Check sheet for the modelled part. Datum: model origin and axes. Units: mm. A direction names the side the tool comes from. Coordinates: 2 decimals unless noted, no trailing zeros. Loops run counter-clockwise (first coordinate to the right, second up) from the corner with the lowest first, then second, coordinate; pieces in that order, holes last.
from build123d import *

# Parameters (mm, degrees)
EXTRUDE_1_DEPTH     = 20
SKETCH_3_R          = 2.1
CUT_EXTRUDE_1_DEPTH = 10
FILLET_1_R          = 8
FILLET_2_R          = 3


with BuildPart() as part:
    # 草图2 → 凸台-拉伸1 (new body)
    with BuildSketch(Plane(origin=(0, 0, 0), x_dir=(1, 0, 0), z_dir=(0, 1, 0))):
        Polygon((0, -7.75), (0, 7.75), (-11, 7.75), (-15, 7.75), (-15, 20), (-15, 24), (-11, 24), (-11, 20), (-11, 11.75), (-7, 11.75), (4, 11.75), (4, -11.75), (-7, -11.75), (-11, -11.75), (-11, -20), (-11, -24), (-15, -24), (-15, -20), (-15, -7.75), (-11, -7.75), align=None)
    extrude(amount=EXTRUDE_1_DEPTH)

    # 草图3 → 切除-拉伸1 (cut)
    with BuildSketch(Plane(origin=(-11, 0, 0), x_dir=(0, 0, -1), z_dir=(1, 0, 0))):
        with Locations((-18, 10)):
            Circle(SKETCH_3_R)
        with Locations((18, 10)):
            Circle(SKETCH_3_R)
    extrude(amount=-CUT_EXTRUDE_1_DEPTH, mode=Mode.SUBTRACT)

    # 圆角1
    fillet_1_edges = [part.edges().sort_by_distance(p)[0] for p in [
        (-13, 0, -24),
        (-13, 0, 24),
        (-13, 20, 24),
        (-13, 20, -24),
    ]]
    fillet(fillet_1_edges, radius=FILLET_1_R)

    # 圆角2
    fillet_2_edges = [part.edges().sort_by_distance(p)[0] for p in [
        (4, 10, -11.75),
        (4, 10, 11.75),
    ]]
    fillet(fillet_2_edges, radius=FILLET_2_R)


solid = part.part
(1) Draft check along Z on faces 1 (the face through (-13.028, 2.281, 21.594)), 2 (the face through (3.1, 10.14, -10.89)), 3 (the face through (-12.972, 10.631, 15.997)). Enter one of: pulls with the +Z half, pulls with the -Z half, needs draft (parallel to the pull), parting line crosses it, or undercut.
(2) Section check B-B, the plane x = -3. Enter the section's corners in (y, z).
(3) Set-up check for faces 4 (the face through (4, 10, 0)), 5 (the face through (-11, 10, -15)), 6 (the face through (-8, 10, -7.75)), 7 (the face through (1, 20, 0)), 8 (the face through (-11, 10, 15)): record each of +Z, -Z, +X, -X, +Y, -Y from which the full face is reachable in a straight line by a thin tool's end or side.
(4) Section check C-C, the plane z = -18. Enter the section's corners in (x, y), plus the area to 3 significant figures.
(5) Section check D-D, the plane y = 14. Enter the section's corners in (x, z), plus the area to 3 significant figures.
(6) Section check A-A, the plane y = 10. Enter the section's corners in (x, z).
(7) Scan lines: line 1 along Z through (x, y) = (-9, 16.5); line 2 along X through (y, z) = (14.5, 6); line 3 along X through (y, z) = (5.75, -20). Record each from-to range of solid material in increasing order.
(8) Gauge pin test, flat ends, axial feed: P1, Ø9.5, axis at x = -6, y = 7, coming from the -Z side; P2, Ø6.5, axis at y = 10, z = 18, coming from the +X side; P3, Ø3.5, axis at x = -5, y = 11.5, coming from the +Z side. Record the tip position at first contact, or that the pin passes through.
Determined:
1. face 1: pulls with the +Z half
1. face 2: pulls with the -Z half
1. face 3: undercut
2. outline: (0, -11.75) - (20, -11.75) - (20, -7.75) - (0, -7.75) - close; (0, 7.75) - (20, 7.75) - (20, 11.75) - (0, 11.75) - close
3. face 4: +Z, -Z, +X, +Y, -Y
3. face 5: -Z, +X, +Y, -Y
3. face 6: -X, +Y, -Y
3. face 7: +Z, -Z, +X, -X, +Y
3. face 8: +Z, +X, +Y, -Y
4. outline: (-15, 0.25) - (-11, 0.25) - (-11, 7.9) - (-15, 7.9) - close; (-15, 12.1) - (-11, 12.1) - (-11, 19.75) - (-15, 19.75) - close
4. area: 61.2 mm2
5. outline: (-15, -23.75) - (-11, -23.75) - (-11, -11.75) - (1, -11.75) arc R3 ccw to (4, -8.75) - (4, 8.75) arc R3 ccw to (1, 11.75) - (-11, 11.75) - (-11, 23.75) - (-15, 23.75) - (-15, 7.75) - (0, 7.75) - (0, -7.75) - (-15, -7.75) - close
5. area: 306 mm2
6. outline: (-15, -24) - (-11, -24) - (-11, -20.1) - (-15, -20.1) - close; (-15, -15.9) - (-11, -15.9) - (-11, -11.75) - (1, -11.75) arc R3 ccw to (4, -8.75) - (4, 8.75) arc R3 ccw to (1, 11.75) - (-11, 11.75) - (-11, 15.9) - (-15, 15.9) - (-15, 7.75) - (0, 7.75) - (0, -7.75) - (-15, -7.75) - close; (-15, 20.1) - (-11, 20.1) - (-11, 24) - (-15, 24) - close
7. line 1: z = -11.75 to -7.75, 7.75 to 11.75
7. line 2: x = 0 to 4
7. line 3: x = -15 to -11
8. P1: stops at z = -11.75
8. P2: stops at x = -11
8. P3: stops at z = 11.75
